Read the model definition and answer for the solid it produces. Units are mm, in the model's axes. A direction names the side the tool comes from. Coordinates: 2 decimals unless noted, no trailing zeros. Order: outer loops, then holes, each group sorted by start corner. A loop starts at its lowest first (then second) coordinate and runs counter-clockwise, first axis right, second up. Notation, with made-up numbers: (-36.75, 67.5) - (0.25, 67.5) arc R32 ccw to (0.25, 96.5) - close; hole circle Ø11 at (23, 24). An arc over 180 degrees is marked (long way). Use one line per item in the form item = value.
```python
from build123d import *

# Parameters (mm, degrees)
SKETCH1_R                = 2.5
SKETCH1_R_2              = 1.5
BOSS_EXTRUDE1_DEPTH      = 74
BOSS_EXTRUDE2_START      = -6
SKETCH2_R                = 3
SKETCH2_R_2              = 1.5
BOSS_EXTRUDE2_DEPTH      = 6
CHAMFER1_SIZE            = 1
CHAMFER1_OF_MIRROR1_SIZE = 1


with BuildPart() as part:
    # Sketch1 → Boss-Extrude1 (new body)
    with BuildSketch(Plane.XY):
        Circle(SKETCH1_R)
        Circle(SKETCH1_R_2, mode=Mode.SUBTRACT)
    extrude(amount=BOSS_EXTRUDE1_DEPTH)

    # Sketch2 → Boss-Extrude2 (add)
    with BuildSketch(Plane.XY.offset(74).offset(BOSS_EXTRUDE2_START)):
        Circle(SKETCH2_R)
        Circle(SKETCH2_R_2, mode=Mode.SUBTRACT)
    boss_extrude2 = extrude(amount=BOSS_EXTRUDE2_DEPTH)

    # Chamfer1
    # the kernel refuses this chamfer: 1 mm, written as the material it takes off along each edge
    with BuildSketch(Plane(origin=(0, 0, 68), x_dir=(1, 0, 0), z_dir=(0, -1, 0))) as chamfer1_piece_1_section:
        Polygon((3 - CHAMFER1_SIZE, 0), (3, CHAMFER1_SIZE), (3, 0), align=None)
    chamfer1_piece_1 = revolve(axis=Axis((0, 0, 68), (0, 0, 1)), mode=Mode.PRIVATE)
    chamfer1_piece_1 = chamfer1_piece_1 - Plane(origin=(0, 0, 68.750504242), x_dir=(1, 0, 0), z_dir=(0, 0, -1)) * Cylinder(2.5, 12, mode=Mode.PRIVATE)
    add(chamfer1_piece_1, mode=Mode.SUBTRACT)

    # Mirror1: Boss-Extrude2 across plane
    add(boss_extrude2.mirror(Plane.XY.offset(37)))

    # Chamfer1 of Mirror1
    # the kernel refuses this chamfer: 1 mm, written as the material it takes off along each edge
    with BuildSketch(Plane(origin=(0, 0, 6), x_dir=(1, 0, 0), z_dir=(0, -1, 0))) as chamfer1_of_mirror1_piece_1_section:
        Polygon((3, -CHAMFER1_OF_MIRROR1_SIZE), (3 - CHAMFER1_OF_MIRROR1_SIZE, 0), (3, 0), align=None)
    chamfer1_of_mirror1_piece_1 = revolve(axis=Axis((0, 0, 6), (0, 0, 1)), mode=Mode.PRIVATE)
    chamfer1_of_mirror1_piece_1 = chamfer1_of_mirror1_piece_1 - Plane(origin=(0, 0, 5.249495758), x_dir=(1, 0, 0), z_dir=(0, 0, -1)) * Cylinder(2.5, 12, mode=Mode.PRIVATE)
    add(chamfer1_of_mirror1_piece_1, mode=Mode.SUBTRACT)


solid = part.part
```
(1) The mould has two halves that part along X. Classify faces 3 (the cylindrical face through (-3, 0, 3)), 4 (the flat face through (1.3, -1.3, 74)), 5 (the cylindrical face through (-1.5, 0.07, 36.48)): +X half, -X half, draft (parallel to the pull), parting line (faces both ways), or undercut.
Answer list:
face_3 = parting line
face_4 = draft
face_5 = undercut
(2) Straight lines are drawn through the part: L1, parallel to X at y = -0.05, z = 22; L2, parallel to Y at x = -1.3, z = 27.5. For each, find the intervals that lie inside material, in ascending order.
Answer list:
L1 = -2.5 to -1.5, 1.5 to 2.5
L2 = -2.14 to -0.75, 0.75 to 2.14
(3) Section A-A, the plane y = 0 is taken. Write down the section's boundary in (x, z), then the cut area to 4 significant figures.
Answer list:
outline = (-3, 0) - (-1.5, 0) - (-1.5, 74) - (-3, 74) - (-3, 69) - (-2.5, 68.5) - (-2.5, 5.5) - (-3, 5) - close; (1.5, 0) - (3, 0) - (3, 5) - (2.5, 5.5) - (2.5, 68.5) - (3, 69) - (3, 74) - (1.5, 74) - close
area = 158.5 mm2
(4) Section C-C, the plane z = 35 is taken. Write down the section's boundary in (x, y), then the cut area to 3 significant figures.
Answer list:
outline = circle Ø5 at (0, 0); hole circle Ø3 at (0, 0)
area = 12.6 mm2
(5) Which of the six approach directions +Z, -Z, +X, -X, +Y, -Y give full straight-line access (tool end or side, diameter ignored) to faces 1 (the cylindrical face through (-3, 0, 71)), 2 (the cylindrical face through (-0.54, 2.44, 36.56))?
Answer list:
face_1 = +Z, -Z
face_2 = none
